```python
from build123d import *

# Parameters (mm, degrees)
BOSS_EXTRUDE1_DEPTH = 3
SKETCH3_W           = 4
SKETCH3_H           = 3
BOSS_EXTRUDE2_DEPTH = 3
SKETCH4_W           = 4
SKETCH4_H           = 3
BOSS_EXTRUDE3_DEPTH = 3
SKETCH5_R           = 1
CUT_EXTRUDE1_DEPTH  = 23.363531015
SKETCH6_R           = 1
CUT_EXTRUDE2_DEPTH  = 23.363531015


with BuildPart() as part:
    # Sketch2 → Boss-Extrude1 (new body)
    with BuildSketch(Plane.XY):
        with BuildLine():
            Line((-11.556982343, -12.333868379), (8.443017657, -12.333868379))
            Line((8.443017657, -12.333868379), (8.443017657, 5.666131621))
            Line((8.443017657, 5.666131621), (-11.556982343, 5.666131621))
            Line((-11.556982343, 5.666131621), (-11.556982343, 3.166131621))
            Line((-11.556982343, 3.166131621), (-2.556982343, 3.166131621))
            ThreePointArc((-2.556982343, 3.166131621), (3.943017657, -3.333868379), (-2.556982343, -9.833868379))
            Line((-2.556982343, -9.833868379), (-11.556982343, -9.833868379))
            Line((-11.556982343, -9.833868379), (-11.556982343, -12.333868379))
        make_face()
    extrude(amount=-BOSS_EXTRUDE1_DEPTH)

    # Sketch3 → Boss-Extrude2 (add)
    with BuildSketch(Plane(origin=(0, 5.666131621, 0), x_dir=(1, 0, 0), z_dir=(0, 1, 0))):
        with Locations((-9.556982343, 1.5)):
            Rectangle(SKETCH3_W, SKETCH3_H)
    extrude(amount=BOSS_EXTRUDE2_DEPTH)

    # Sketch4 → Boss-Extrude3 (add)
    with BuildSketch(Plane.XZ.offset(12.333868379)):
        with Locations((-9.556982343, -1.5)):
            Rectangle(SKETCH4_W, SKETCH4_H)
    extrude(amount=BOSS_EXTRUDE3_DEPTH)

    # Sketch5 → Cut-Extrude1 (cut, through all)
    with BuildSketch(Plane(origin=(-7.556982343, 0, 0), x_dir=(0, 0, -1), z_dir=(1, 0, 0))):
        with Locations((1.5, 7.166131621)):
            Circle(SKETCH5_R)
    extrude(amount=-CUT_EXTRUDE1_DEPTH, mode=Mode.SUBTRACT)

    # Sketch6 → Cut-Extrude2 (cut, through all)
    with BuildSketch(Plane(origin=(-7.556982343, 0, 0), x_dir=(0, 0, -1), z_dir=(1, 0, 0))):
        with Locations((1.5, -13.833868379)):
            Circle(SKETCH6_R)
    extrude(amount=-CUT_EXTRUDE2_DEPTH, mode=Mode.SUBTRACT)


solid = part.part
```
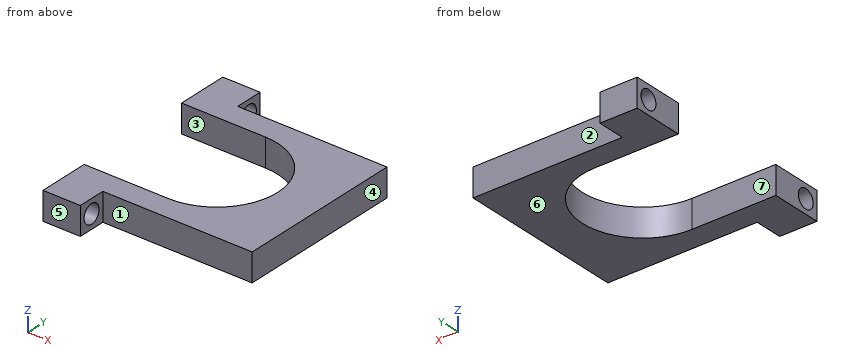
Source: CAD feature listing. Evaluate the final solid. Frame: model axes, mm. Face numbers are marked on the shaded views. A direction names the side the tool comes from. Round coordinates to 2 decimals unless told otherwise and drop trailing zeros. Loops run counter-clockwise (first coordinate to the right, second up) from the corner with the lowest first, then second, coordinate; pieces in that order, holes last.
(1) Contact query for flat-ended pins moving along their axis: pin 1 Ø0.9 at (x, z) = (-3.5, -2) entering from +Y; pin 2 Ø1.5 at (y, z) = (7.5, -1.5) entering from +X; pin 3 Ø1 at (x, z) = (-5.5, -1.5) entering from -Y; pin 4 Ø1.6 at (y, z) = (-13.83, -1.5) entering from +X. Output: stop coordinate, or through.
From the geometry:
pin 1: stops at y = 5.67
pin 2: stops at x = -7.56
pin 3: stops at y = -12.33
pin 4: passes through
(2) Section query A-A (z = -1.5). Output: boundary loops of the cut face in (x, y), and give its area (3 significant figures).
From the geometry:
outline: (-11.56, -15.33) - (-7.56, -15.33) - (-7.56, -14.83) - (-11.56, -14.83) - close; (-11.56, -12.83) - (-7.56, -12.83) - (-7.56, -12.33) - (8.44, -12.33) - (8.44, 5.67) - (-7.56, 5.67) - (-7.56, 6.17) - (-11.56, 6.17) - (-11.56, 3.17) - (-2.56, 3.17) arc R6.5 cw to (-2.56, -9.83) - (-11.56, -9.83) - close; (-11.56, 8.17) - (-7.56, 8.17) - (-7.56, 8.67) - (-11.56, 8.67) - close
area: 185 mm2
(3) Access query for the marked faces 1, 2, 3 and 4. Directions: +Z, -Z, +X, -X, +Y, -Y. A direction counts if a zero-diameter tool reaches every point of the face in a straight line with its end or side. Return the directions, or none.
From the geometry:
face 1: +Z, -Z, +X, -Y
face 2: +Z, -Z, +X, +Y
face 3: +Z, -Z, -X
face 4: +Z, -Z, +X, +Y, -Y
(4) Section query D-D (y = -3.5). Output: boundary loops of the cut face in (x, z).
From the geometry:
outline: (3.94, -3) - (8.44, -3) - (8.44, 0) - (3.94, 0) - close
(5) Pull-direction query (Y, two-part tool) for the marked faces 5, 6 and 7; classes: +Y half, -Y half, draft (parallel to the pull), parting line (faces both ways), or undercut.
From the geometry:
face 5: -Y half
face 6: draft
face 7: undercut
(6) Section query B-B (x = 2). Output: boundary loops of the cut face in (y, z).
From the geometry:
outline: (-12.33, -3) - (-7.97, -3) - (-7.97, 0) - (-12.33, 0) - close; (1.3, -3) - (5.67, -3) - (5.67, 0) - (1.3, 0) - close
(7) Section query C-C (y = 2.75). Output: boundary loops of the cut face in (x, z).
From the geometry:
outline: (-0.27, -3) - (8.44, -3) - (8.44, 0) - (-0.27, 0) - close
(8) Material intervals for probe 1 along Y at (x, z) = (-8.8, -1.5); probe 2 along Y at (x, z) = (-3.75, -2.5); probe 3 along X at (y, z) = (6.25, -0.1), sorted ascending.
From the geometry:
probe 1: y = -15.33 to -14.83, -12.83 to -9.83, 3.17 to 6.17, 8.17 to 8.67
probe 2: y = -12.33 to -9.83, 3.17 to 5.67
probe 3: x = -11.56 to -7.56
